For this review, take the finished solid that the model builds, in its own axes (mm). A direction names the side the tool comes from. Round coordinates to 2 decimals unless told otherwise and drop trailing zeros. Write each loop counter-clockwise with the first axis right and the second up, starting at its lowest first coordinate (ties: lowest second). Pieces come first, ordered by that corner, then holes. Notation, with made-up numbers: (74, 70.5) -> (91, 70.5) arc R12 ccw to (91, 93.5) -> close; hole circle Ø10 at (74.25, -28). An arc over 180 degrees is marked (long way). Answer in a Markdown table with one row per item.
Autodesk Fusion 360 part; units mm, degrees
sketch "Sketch1" plane through (0, 0, 0) normal (0, 1, 0) x (1, 0, 0)
  line L0 (25, -12.5) -> (-25, -12.5)
  line L1 (-25, -12.5) -> (-25, 12.5)
  line L2 (-25, 12.5) -> (25, 12.5)
  line L3 (25, 12.5) -> (25, -12.5)
  line L4 (25, -12.5) -> (-25, 12.5) construction
  line L5 (-25, -12.5) -> (25, 12.5) construction
  dimension "d1" = 50
  dimension "d2" = 25
extrude "Extrude1" add sketch "Sketch1" along normal blind 30 makes body 1
sketch "Sketch2" plane through (0, 30, 0) normal (0, 1, 0) x (-1, 0, 0)
  line L0 (-25, -12.5) -> (25, -12.5)
  line L1 (25, -12.5) -> (25, 12.5)
  line L2 (25, 12.5) -> (-25, 12.5)
  line L3 (-25, 12.5) -> (-25, -12.5)
  circle A0 centre (0, 0) radius 10
  dimension "d5" = 20
extrude "Extrude2" add sketch "Sketch2" along normal blind 25 contours A0 bodies 1
sketch "Sketch3" plane through (0, 0, 0) normal (0, -1, 0) x (1, 0, 0)
  line L0 (-25, -12.5) -> (25, -12.5)
  line L1 (25, -12.5) -> (25, 12.5)
  line L2 (25, 12.5) -> (-25, 12.5)
  line L3 (-25, 12.5) -> (-25, -12.5)
  line L4 (11, -3) -> (-11, -3)
  line L5 (-11, -3) -> (-11, 3)
  line L6 (-11, 3) -> (11, 3)
  line L7 (11, 3) -> (11, -3)
  line L8 (11, -3) -> (-11, 3) construction
  line L9 (-11, -3) -> (11, 3) construction
  dimension "d8" = 22
  dimension "d9" = 6
extrude "Extrude4" add sketch "Sketch3" along normal blind 10 contours L4 L5 L6 L7 bodies 1
sketch "Sketch4" plane through (0, 0, 3) normal (0, 0, 1) x (1, 0, 0)
  line L0 (11, 0) -> (-11, 0)
  line L1 (-11, 0) -> (-11, -10)
  line L2 (-11, -10) -> (11, -10)
  line L3 (11, -10) -> (11, 0)
  circle A0 centre (-6, -7) radius 1.5
  circle A1 centre (6, -7) radius 1.5
  dimension "d16" = 3
  dimension "d19" = 3
extrude "Extrude5" cut sketch "Sketch4" against normal blind 15 contours A0 | A1 bodies 1
extrude "Extrude3" add sketch "Sketch3" along normal blind 15 contours L4 L5 L6 L7 bodies 1
sketch "Sketch5" plane through (0, 0, 3) normal (0, 0, 1) x (1, 0, 0)
  line L0 (11, 0) -> (-11, 0)
  line L1 (-11, 0) -> (-11, -15)
  line L2 (-11, -15) -> (11, -15)
  line L3 (11, -15) -> (11, 0)
  circle A0 centre (-6, -12) radius 1.5
  circle A1 centre (6, -12) radius 1.5
  dimension "d26" = 3
  dimension "d27" = 3
extrude "Extrude6" cut sketch "Sketch5" against normal blind 21 contours A0 | A1 bodies 1
copy_body "Body->Comp2" bodies 1 removing the originals makes body 2 in component "Component"
component "Component" placed x (1, 0, 0) y (0, 1, 0) z (0, 0, 1) at (0, 0, 0)
1) Consider section B-B on y = -12. State the section outline as (x, z) points.
Solved:
| item | result |
|---|---|
| outline | (-11, -3) -> (-7.5, -3) -> (-7.5, 3) -> (-11, 3) -> close; (-4.5, -3) -> (4.5, -3) -> (4.5, 3) -> (-4.5, 3) -> close; (7.5, -3) -> (11, -3) -> (11, 3) -> (7.5, 3) -> close |
2) Consider section D-D on x = 0. State the section outline as (y, z) points, then the cut area to 3 significant figures.
Solved:
| item | result |
|---|---|
| outline | (-15, -3) -> (0, -3) -> (0, -12.5) -> (30, -12.5) -> (30, -10) -> (55, -10) -> (55, 10) -> (30, 10) -> (30, 12.5) -> (0, 12.5) -> (0, 3) -> (-15, 3) -> close |
| area | 1,340 mm² |
3) Clearance check with flat-ended pins moving along their axes: pin 1 Ø1.8 at (x, y) = (6, -12) entering from +Z; pin 2 Ø3 at (y, z) = (42, 0.5) entering from +X; pin 3 Ø5 at (y, z) = (-8.5, 1) entering from -X; pin 4 Ø1 at (x, z) = (-14, 2) entering from +Y. State where each tip first meets the part, or that it passes through.
Solved:
| item | result |
|---|---|
| pin 1 | through |
| pin 2 | x = 10 |
| pin 3 | x = -11 |
| pin 4 | y = 30 |
4) Mouldability with a two-part tool opening along Y and no side actions: class faces 5 (the flat face through (0, -15, 0)), 6 (the flat face through (0, 15, 12.5)), 7 (the cylindrical face through (-7.2, -12.9, 0)) as pulls with the +Y half, pulls with the -Y half, needs draft (parallel to the pull), parting line crosses it, or undercut.
Solved:
| item | result |
|---|---|
| face 5 | pulls with the -Y half |
| face 6 | needs draft |
| face 7 | undercut |
5) Consider section A-A on x = -6. State the section outline as (y, z) points.
Solved:
| item | result |
|---|---|
| outline | (-15, -3) -> (-13.5, -3) -> (-13.5, 3) -> (-15, 3) -> close; (-10.5, -3) -> (0, -3) -> (0, -12.5) -> (30, -12.5) -> (30, -8) -> (55, -8) -> (55, 8) -> (30, 8) -> (30, 12.5) -> (0, 12.5) -> (0, 3) -> (-10.5, 3) -> close |
6) For line 1 (Y direction, x = -6, z = -0.2); line 2 (Y direction, x = -3, z = -4.5); line 3 (Y direction, x = 17.5, z = -11), list the stretches that pass through material, from the lowest coordinate up. Write a range as [from, to].
Solved:
| item | result |
|---|---|
| line 1 | [-15, -13.5], [-10.5, 55] |
| line 2 | [0, 55] |
| line 3 | [0, 30] |
7) For faces 1 (the flat face through (11, -7, 0)), 2 (the flat face through (0, -7, -3)), 3 (the flat face through (0, -7, 3)), 4 (the cylindrical face through (2.17, 42.32, 9.76)), list the 3-axis set-ups (+Z, -Z, +X, -X, +Y, -Y) from which the entire face can be reached by the end or side of a thin tool; tool diameter is ignored.
Solved:
| item | result |
|---|---|
| face 1 | +Z, -Z, +X, -Y |
| face 2 | -Z, +X, -X, -Y |
| face 3 | +Z, +X, -X, -Y |
| face 4 | +Y |
8) Consider section C-C on z = 0. State the section outline as (x, y) points.
Solved:
| item | result |
|---|---|
| outline | (-25, 0) -> (-11, 0) -> (-11, -15) -> (11, -15) -> (11, 0) -> (25, 0) -> (25, 30) -> (10, 30) -> (10, 55) -> (-10, 55) -> (-10, 30) -> (-25, 30) -> close; hole circle Ø3 at (-6, -12); hole circle Ø3 at (6, -12) |
